Here's the drawing with two shaded views (mm, measured from the low corner). I have some questions. Coordinates: 2 decimals unless noted, no trailing zeros. Order: outer loops, then holes, each group sorted by start corner. A loop starts at its lowest first (then second) coordinate and runs counter-clockwise, first axis right, second up. Notation, with made-up numbers: (0.5, -15.5) -> (45.5, -15.5) arc R34 ccw to (45.5, 19.5) -> close; hole circle Ø6 at (-25.5, -28.5). An arc over 180 degrees is marked (long way). Answer in a Markdown table with one row per item. Add a question column.
1. Will these pins go through, and if not, where does the flat tip stop? pin 1 (1.4 mm diameter, centred on x = 3.67, y = 3.18, fed in from +Z); pin 2 (1 mm diameter, centred on y = 0.5, z = 6, fed in from -X) (1 decimal); pin 3 (2.5 mm diameter, centred on x = 3.67, y = 3.18, fed in from +Z); pin 4 (1 mm diameter, centred on y = 5.5, z = 2.5, fed in from +X).
2. Imagine slicing it at D-D on y = 5. Write out the boundary of the cut face in (x, z), plus the area to 3 significant figures.
3. If I drill on line 1 along X through (y, z) = (4, 20.5) (1 decimal); line 2 along X through (y, z) = (3, 22.5); line 3 along X through (y, z) = (1.75, 6.25), over which ranges is the centre line in solid material (lowest first)? Write a range as [from, to].
4. Imagine slicing it at C-C on x = 6.5. Write out the boundary of the cut face in (y, z).
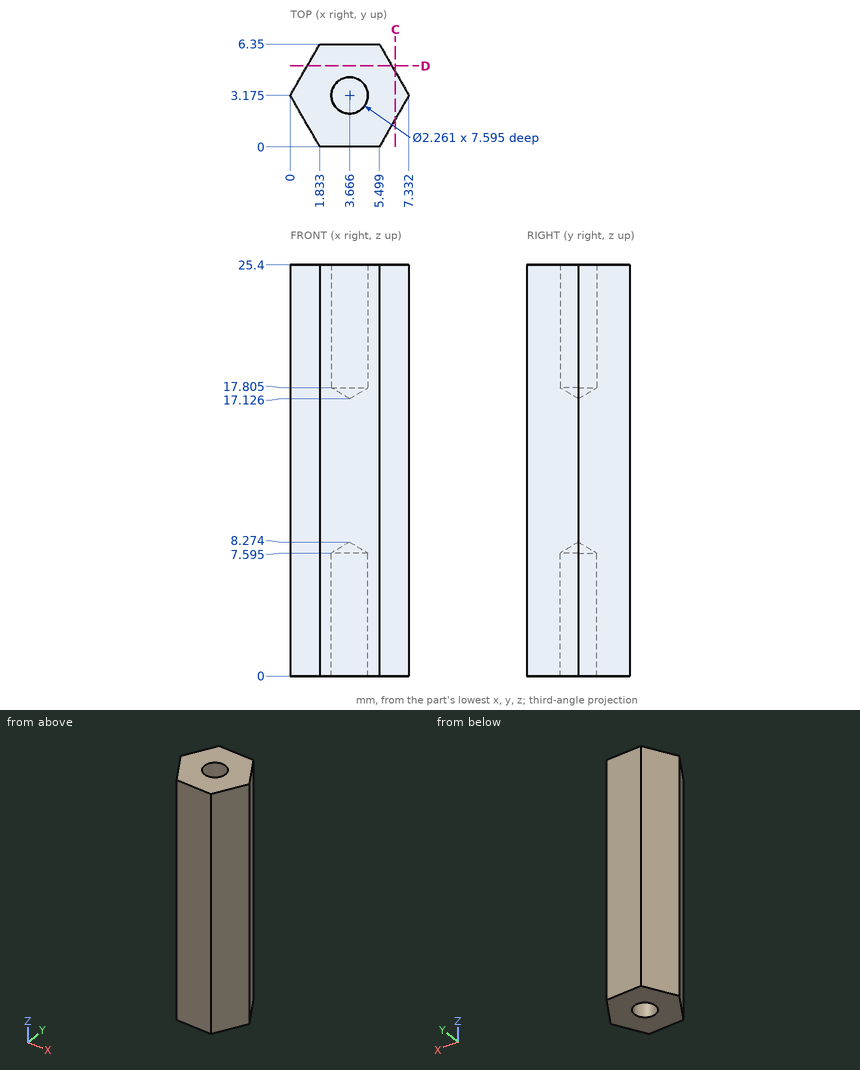
Answers follow:
| question | item | result |
|---|---|---|
| 1 | pin 1 | stops at z = 17.55 |
| 1 | pin 2 | stops at x = 1.3 |
| 1 | pin 3 | stops at z = 25.4 |
| 1 | pin 4 | stops at x = 6.28 |
| 2 | outline | (1.05, 0) -> (6.28, 0) -> (6.28, 25.4) -> (1.05, 25.4) -> close |
| 2 | area | 133 mm² |
| 3 | line 1 | x = [0.5, 2.9], [4.4, 6.9] |
| 3 | line 2 | x = [0.1, 2.55], [4.78, 7.23] |
| 3 | line 3 | x = [0.82, 6.51] |
| 4 | outline | (1.73, 0) -> (4.62, 0) -> (4.62, 25.4) -> (1.73, 25.4) -> close |
